from build123d import *

# Parameters (mm, degrees)
SKETCH1_R           = 3.25
BOSS_EXTRUDE1_DEPTH = 5
CHAMFER2_SIZE       = 0.25


with BuildPart() as part:
    # Sketch1 → Boss-Extrude1 (new body)
    with BuildSketch(Plane(origin=(0, 0, 0), x_dir=(1, 0, 0), z_dir=(0, 1, 0))):
        Polygon((-3.75277675, -6.5), (3.75277675, -6.5), (7.505553499, 0), (3.75277675, 6.5), (-3.75277675, 6.5), (-7.505553499, 0), align=None)
        Circle(SKETCH1_R, mode=Mode.SUBTRACT)
    extrude(amount=BOSS_EXTRUDE1_DEPTH)

    # Sketch2 → Cut-Revolve1 (revolve, cut)
    with BuildSketch(Plane(origin=(0, 0, 0), x_dir=(0, 0, -1), z_dir=(1, 0, 0))):
        Polygon((6.5, 5), (7.55, 6.05), (7.55, 3.95), align=None)
        Polygon((7.55, 1.05), (6.5, 0), (7.55, -1.05), align=None)
    revolve(axis=Axis((0, 5, 0), (0, -1, 0)), mode=Mode.SUBTRACT)

    # Chamfer2
    chamfer2_edges = [part.edges().sort_by_distance(p)[0] for p in [
        (-3.25, 0, 0),
        (-3.25, 5, 0),
    ]]
    chamfer(chamfer2_edges, length=CHAMFER2_SIZE)


solid = part.part
Part model, mm, in its own coordinate system. Give positions to 0.01 mm unless a question says otherwise; leave off trailing zeros. Write each loop counter-clockwise with the first axis right and the second up, starting at its lowest first coordinate (ties: lowest second). Pieces come first, ordered by that corner, then holes.
1) Two-plate mould, pull along Z, no slides. Class faces 1 (the face through (-5.66, 2.46, 3.2)), 2 (the face through (-3.38, 4.76, -5.83)), 3 (the face through (-2.579, 2.468, 1.978)): released by +Z, released by -Z, zero draft, split by the parting line, or undercut.
Resolved:
face 1: released by +Z
face 2: released by -Z
face 3: undercut
2) Probe L1, parallel to Z at x = 0, y = 1.75; L2, parallel to X at y = 2.4, z = 2; L3, parallel to X at y = 2.6, z = -1.75. List the from-to ranges inside material, lowest first.
Resolved:
L1: z = -6.5 to -3.25, 3.25 to 6.5
L2: x = -6.35 to -2.56, 2.56 to 6.35
L3: x = -6.5 to -2.74, 2.74 to 6.5
3) Pin check, flat tips, straight feed: pin 1 (3 mm diameter, centred on x = 2.5, z = 0.5, fed in from -Y); pin 2 (1 mm diameter, centred on y = 3.5, z = 2, fed in from +X); pin 3 (3 mm diameter, centred on y = 2, z = 5, fed in from -X). Stop position of each tip, or through.
Resolved:
pin 1: stops at y = 0
pin 2: stops at x = 6.64
pin 3: stops at x = -5.48
4) Cut at A-A on y = 2.45. Write the cut outline in (x, z).
Resolved:
outline: (-7.51, 0) - (-3.75, -6.5) - (3.75, -6.5) - (7.51, 0) - (3.75, 6.5) - (-3.75, 6.5) - close; hole circle Ø6.5 at (0, 0)
5) Cut at B-B on y = 4.5. Write the cut outline in (x, z), then the cut area to 3 significant figures.
Resolved:
outline: (-6.93, -1) - (-4.33, -5.5) arc R7 ccw to (-2.6, -6.5) - (2.6, -6.5) arc R7 ccw to (4.33, -5.5) - (6.93, -1) arc R7 ccw to (6.93, 1) - (4.33, 5.5) arc R7 ccw to (2.6, 6.5) - (-2.6, 6.5) arc R7 ccw to (-4.33, 5.5) - (-6.93, 1) arc R7 ccw to start; hole circle Ø6.5 at (0, 0)
area: 110 mm2
